```python
from build123d import *

# Parameters (mm, degrees)
SKETCH1_W                     = 110
SKETCH1_H                     = 37
BOSS_EXTRUDE1_DEPTH           = 5
M2_CLEARANCE_HOLE1_AT_2_COUNT = 2
M2_CLEARANCE_HOLE1_AT_2_PITCH = 27
SKETCH5_W                     = 2
SKETCH5_H                     = 5
CUT_EXTRUDE1_DEPTH            = 4
SKETCH6_W                     = 19.5
SKETCH6_H                     = 12.5
CUT_EXTRUDE2_DEPTH            = 10
CUT_EXTRUDE3_DEPTH            = 59.243025334


with BuildPart() as part:
    # Sketch1 → Boss-Extrude1 (new body)
    with BuildSketch(Plane.XY):
        Rectangle(SKETCH1_W, SKETCH1_H)
    extrude(amount=BOSS_EXTRUDE1_DEPTH)

    # Sketch4 → M2 Clearance Hole1 (revolve, cut)
    with BuildSketch(Plane(origin=(-55, 13.5, 2.5), x_dir=(0, 0, 1), z_dir=(0, 1, 0))):
        Polygon((0, 0), (0, 14.721032743), (1.2, 14), (1.2, 0), align=None)
    m2_clearance_hole1 = revolve(axis=Axis((-61.35, 13.5, 2.5), (1, 0, 0)), mode=Mode.SUBTRACT)

    # M2 Clearance Hole1 at 2: M2 Clearance Hole1 ×2
    with Locations(*[(0, -i * M2_CLEARANCE_HOLE1_AT_2_PITCH, 0) for i in range(1, M2_CLEARANCE_HOLE1_AT_2_COUNT)]):
        add(m2_clearance_hole1, mode=Mode.SUBTRACT)

    # Sketch5 → Cut-Extrude1 (cut)
    with BuildSketch(Plane.XY.offset(5)):
        with Locations((-40.9, 13.5)):
            Rectangle(SKETCH5_W, SKETCH5_H)
        with Locations((-40.9, -13.5)):
            Rectangle(SKETCH5_W, SKETCH5_H)
    cut_extrude1 = extrude(amount=-CUT_EXTRUDE1_DEPTH, mode=Mode.SUBTRACT)

    # Mirror1: M2 Clearance Hole1, Cut-Extrude1 across plane
    add(m2_clearance_hole1.mirror(Plane(origin=(0, 0, 0), x_dir=(0, 0, 1), z_dir=(1, 0, 0))), mode=Mode.SUBTRACT)
    add(cut_extrude1.mirror(Plane(origin=(0, 0, 0), x_dir=(0, 0, 1), z_dir=(1, 0, 0))), mode=Mode.SUBTRACT)

    # Mirror1 copy 1 sketch → Mirror1 copy 1 (revolve, cut)
    with BuildSketch(Plane(origin=(55, -13.5, 2.5), x_dir=(0, 0, 1), z_dir=(0, 1, 0))):
        Polygon((0, 0), (0, -14.721032743), (1.2, -14), (1.2, 0), align=None)
    revolve(axis=Axis((61.35, -13.5, 2.5), (1, 0, 0)), mode=Mode.SUBTRACT)

    # Sketch6 → Cut-Extrude2 (cut)
    with BuildSketch(Plane.XY.offset(5)):
        with Locations((41.25, -2.25)):
            Rectangle(SKETCH6_W, SKETCH6_H)
    extrude(amount=-CUT_EXTRUDE2_DEPTH, mode=Mode.SUBTRACT)

    # Sketch7 → Cut-Extrude3 (cut, through all)
    with BuildSketch(Plane.XY.offset(5)):
        Polygon((-34.9, -3), (-34.9, -13.5), (17.424359974, -13.5), (-23.127364164, -3), align=None)
        Polygon((-34.9, 13.5), (-34.9, 3), (-25.872635836, 3), (25.310097731, -10.252672084), (26.9, -8.878654338), (26.9, 13.5), align=None)
    extrude(amount=-CUT_EXTRUDE3_DEPTH, mode=Mode.SUBTRACT)


solid = part.part
```
Design review of the part built by this model. Coordinates are the model's own, in mm. A direction names the side the tool comes from. Give positions to 0.01 mm unless a question says otherwise; leave off trailing zeros. Order: outer loops, then holes, each group sorted by start corner. A loop starts at its lowest first (then second) coordinate and runs counter-clockwise, first axis right, second up. Notation, with made-up numbers: (-35, -6) - (-1, -6) arc R21 ccw to (-1, 17) - close; hole circle Ø9 at (-10, 24.5). An arc over 180 degrees is marked (long way). Use a Markdown table: item, result. Add a question column.
(1) Add section C-C on z = 2.5. Give the number of separate pieces and of enclosed holes in the cut face, then the cut area to 3 significant figures.
(2) Add section A-A on x = -29. Give the boundary of the cut face in (y, z), then the cut area to 3 significant figures.
(3) Mouldability with a two-part tool opening along Y and no side actions: class faces 1 (the face through (-1, -4, 0)), 2 (the face through (-41, -13, 1)), 3 (the face through (-1, -18.5, 2)) as +Y half, -Y half, draft (parallel to the pull), parting line (faces both ways), or undercut.
(4) Clearance check with flat-ended pins moving along their axes: P1, Ø3, axis at y = 12.5, z = 2.5, coming from the +X side; P2, Ø1, axis at x = 40.5, y = -13.5, coming from the +Z side. State where each tip first meets the part, or that it passes through.
(5) Add section D-D on x = -16.5. Give the boundary of the cut face in (y, z), then the cut area to 3 significant figures.
(6) Add section B-B on y = -6. Give the boundary of the cut face in (x, z), then the cut area to 3 significant figures.
(7) Wall thickness on probe 1 along X at (y, z) = (-15, 4.1); probe 2 along Y at (x, z) = (48.5, 2.5); probe 3 along Y at (x, z) = (-47, 2.5): over which ranges is each line inside the solid? List them lowest first. Write a range as [from, to].
(8) Machinability: for faces 4 (the face through (55, 0, 2)), 5 (the face through (41, 16, 3)), 6 (the face through (-29, -3, 3)), 7 (the face through (48.54, -12.33, 2.24)), which of the approach directions +Z, -Z, +X, -X, +Y, -Y give a long, thin tool a straight path to every point of the face, cutting with its end or side? Answer none if there is none.
Report:
| question | item | result |
|---|---|---|
| 1 | separate pieces | 1 |
| 1 | enclosed holes | 3 |
| 1 | area | 2,320 mm² |
| 2 | outline | (-18.5, 0) - (-13.5, 0) - (-13.5, 5) - (-18.5, 5) - close; (-3, 0) - (3, 0) - (3, 5) - (-3, 5) - close; (13.5, 0) - (18.5, 0) - (18.5, 5) - (13.5, 5) - close |
| 2 | area | 80.0 mm² |
| 3 | face 1 | draft |
| 3 | face 2 | undercut |
| 3 | face 3 | -Y half |
| 4 | P1 | stops at x = 55 |
| 4 | P2 | stops at z = 1 |
| 5 | outline | (-18.5, 0) - (-13.5, 0) - (-13.5, 5) - (-18.5, 5) - close; (-4.72, 0) - (0.57, 0) - (0.57, 5) - (-4.72, 5) - close; (13.5, 0) - (18.5, 0) - (18.5, 5) - (13.5, 5) - close |
| 5 | area | 76.4 mm² |
| 6 | outline | (-55, 0) - (-34.9, 0) - (-34.9, 5) - (-55, 5) - close; (-11.54, 0) - (8.89, 0) - (8.89, 5) - (-11.54, 5) - close; (26.9, 0) - (31.5, 0) - (31.5, 5) - (26.9, 5) - close; (51, 0) - (55, 0) - (55, 5) - (51, 5) - close |
| 6 | area | 246 mm² |
| 7 | probe 1 | x = [-55, -41.9], [-39.9, 39.9], [41.9, 55] |
| 7 | probe 2 | y = [-18.5, -14.7], [-12.3, -8.5], [4, 12.3], [14.7, 18.5] |
| 7 | probe 3 | y = [-18.5, -14.7], [-12.3, 12.3], [14.7, 18.5] |
| 8 | face 4 | +Z, -Z, +X, +Y, -Y |
| 8 | face 5 | +Z |
| 8 | face 6 | +Z, -Z |
| 8 | face 7 | +X |
